```python
from build123d import *

# Parameters (mm, degrees)
SKETCH1_R           = 7
SKETCH1_R_2         = 2.5
BOSS_EXTRUDE1_DEPTH = 5
SKETCH2_R           = 5.25
SKETCH2_R_2         = 4
CUT_EXTRUDE1_DEPTH  = 0.5
CUT_EXTRUDE2_START  = -0.5
SKETCH3_R           = 5.25
SKETCH3_R_2         = 4
CUT_EXTRUDE2_DEPTH  = 0.5
CHAMFER1_SIZE       = 0.3


with BuildPart() as part:
    # Sketch1 → Boss-Extrude1 (new body)
    with BuildSketch(Plane.XY):
        Circle(SKETCH1_R)
        Circle(SKETCH1_R_2, mode=Mode.SUBTRACT)
    extrude(amount=BOSS_EXTRUDE1_DEPTH)

    # Sketch2 → Cut-Extrude1 (cut)
    with BuildSketch(Plane.XY.offset(5)):
        Circle(SKETCH2_R)
        Circle(SKETCH2_R_2, mode=Mode.SUBTRACT)
    extrude(amount=-CUT_EXTRUDE1_DEPTH, mode=Mode.SUBTRACT)

    # Sketch3 → Cut-Extrude2 (cut)
    with BuildSketch(Plane(origin=(0, 0, 0), x_dir=(-1, 0, 0), z_dir=(0, 0, -1)).offset(CUT_EXTRUDE2_START)):
        with Locations(Location((0, 0, 0), (0, 0, 180))):
            Circle(SKETCH3_R)
        with Locations(Location((0, 0, 0), (0, 0, 180))):
            Circle(SKETCH3_R_2, mode=Mode.SUBTRACT)
    extrude(amount=CUT_EXTRUDE2_DEPTH, mode=Mode.SUBTRACT)

    # Chamfer1
    chamfer1_edges = [part.edges().sort_by_distance(p)[0] for p in [
        (-7, 0, 0),
        (-7, 0, 5),
    ]]
    chamfer(chamfer1_edges, length=CHAMFER1_SIZE)


solid = part.part
```
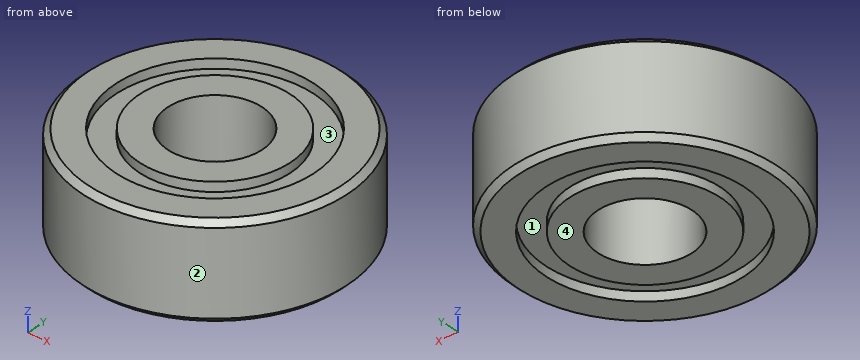
Verification items for the finished model (mm, model axes). Face numbers are marked on the shaded views. Coordinates: 2 decimals unless noted, no trailing zeros. Loops run counter-clockwise (first coordinate to the right, second up) from the corner with the lowest first, then second, coordinate; pieces in that order, holes last. Notation, with made-up numbers: (20, -13) - (25, -13) arc R22 ccw to (25, 21) - close; hole circle Ø11 at (9.25, -6). An arc over 180 degrees is marked (long way). Put each result on its own line as item: value.
Item 1: Section check A-A (x = 0). Enter the section's corners in (y, z), then the cut area to 3 significant figures.
Conclusion:
outline: (-7, 0.3) - (-6.7, 0) - (-5.25, 0) - (-5.25, 0.5) - (-4, 0.5) - (-4, 0) - (-2.5, 0) - (-2.5, 5) - (-4, 5) - (-4, 4.5) - (-5.25, 4.5) - (-5.25, 5) - (-6.7, 5) - (-7, 4.7) - close; (2.5, 0) - (4, 0) - (4, 0.5) - (5.25, 0.5) - (5.25, 0) - (6.7, 0) - (7, 0.3) - (7, 4.7) - (6.7, 5) - (5.25, 5) - (5.25, 4.5) - (4, 4.5) - (4, 5) - (2.5, 5) - close
area: 42.3 mm2
Item 2: Section check C-C (z = 0.7). Enter the section's corners in (x, y).
Conclusion:
outline: circle Ø14 at (0, 0); hole circle Ø5 at (0, 0)
Item 3: Gauge pin test, flat ends, axial feed: pin 1 Ø2 at (y, z) = (-2, 2) entering from -X; pin 2 Ø2 at (y, z) = (-5.5, 3) entering from -X; pin 3 Ø1.5 at (x, z) = (4.5, 1) entering from -Y. Record the tip position at first contact, or that the pin passes through.
Conclusion:
pin 1: stops at x = -6.93
pin 2: stops at x = -5.36
pin 3: stops at y = -5.91
Item 4: Scan lines: line 1 along Y through (x, z) = (0, 0.45); line 2 along Y through (x, z) = (0, 1.5); line 3 along X through (y, z) = (1, 4.6). Record each from-to range of solid material in increasing order.
Conclusion:
line 1: y = -7 to -5.25, -4 to -2.5, 2.5 to 4, 5.25 to 7
line 2: y = -7 to -2.5, 2.5 to 7
line 3: x = -6.93 to -5.15, -3.87 to -2.29, 2.29 to 3.87, 5.15 to 6.93
Item 5: Draft check along Y on the marked faces 1, 2, 3 and 4. Enter one of: pulls with the +Y half, pulls with the -Y half, needs draft (parallel to the pull), parting line crosses it, or undercut.
Conclusion:
face 1: undercut
face 2: parting line crosses it
face 3: undercut
face 4: needs draft
